Verification items for the finished model (mm, model axes). Face numbers are marked on the shaded views. Round coordinates to 2 decimals unless told otherwise and drop trailing zeros. Write each loop counter-clockwise with the first axis right and the second up, starting at its lowest first coordinate (ties: lowest second). Pieces come first, ordered by that corner, then holes.
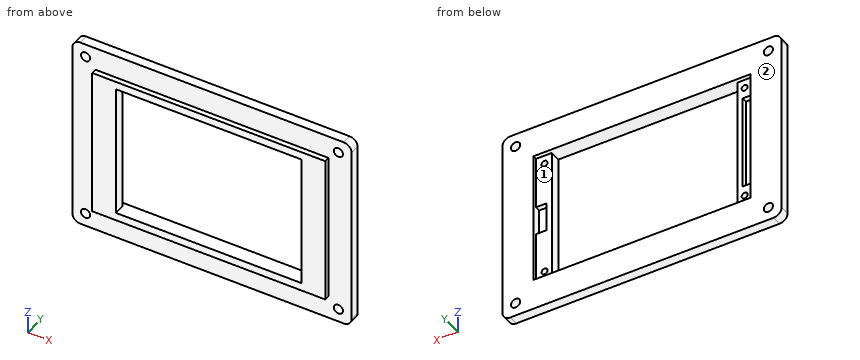
from build123d import *

# Parameters (mm, degrees)
SKETCH_1_W          = 106
SKETCH_1_H          = 74
EXTRUDE_1_DEPTH     = 5.7
SKETCH_2_W          = 70.5
SKETCH_2_H          = 50.5
CUT_EXTRUDE_1_DEPTH = 130.400502317
SKETCH_3_W          = 82.5
SKETCH_3_H          = 50.5
CUT_EXTRUDE_2_DEPTH = 1.6
SKETCH_4_W          = 4
SKETCH_4_H          = 11
SKETCH_4_H_2        = 36
CUT_EXTRUDE_3_DEPTH = 2
SKETCH_5_R          = 1.15
CUT_EXTRUDE_4_DEPTH = 3.9
CUT_EXTRUDE_START   = -5.7
SKETCH_6_W          = 131.135040239
SKETCH_6_H          = 88.560038322
SKETCH_6_W_2        = 88.5
SKETCH_6_H_2        = 56.5
CUT_EXTRUDE_5_DEPTH = 2
SKETCH_7_R          = 1.75
CUT_EXTRUDE_6_DEPTH = 130.32783923
FILLET_1_R          = 3


with BuildPart() as part:
    # Эскиз1 → Бобышка-Вытянуть1 (new body)
    with BuildSketch(Plane(origin=(0, 0, 0), x_dir=(1, 0, 0), z_dir=(0, 1, 0))):
        with Locations((53, 37)):
            Rectangle(SKETCH_1_W, SKETCH_1_H)
    extrude(amount=EXTRUDE_1_DEPTH)

    # Эскиз2 → Вырез-Вытянуть1 (cut, through all)
    with BuildSketch(Plane(origin=(0, 5.7, 0), x_dir=(1, 0, 0), z_dir=(0, 1, 0))):
        with Locations((53, 37)):
            Rectangle(SKETCH_2_W, SKETCH_2_H)
    extrude(amount=-CUT_EXTRUDE_1_DEPTH, mode=Mode.SUBTRACT)

    # Эскиз3 → Вырез-Вытянуть2 (cut)
    with BuildSketch(Plane(origin=(0, 5.7, 0), x_dir=(1, 0, 0), z_dir=(0, 1, 0))):
        with Locations((53, 37)):
            Rectangle(SKETCH_3_W, SKETCH_3_H)
    extrude(amount=-CUT_EXTRUDE_2_DEPTH, mode=Mode.SUBTRACT)

    # Эскиз4 → Вырез-Вытянуть3 (cut)
    with BuildSketch(Plane(origin=(0, 4.1, 0), x_dir=(1, 0, 0), z_dir=(0, 1, 0))):
        with Locations((92.25, 37)):
            Rectangle(SKETCH_4_W, SKETCH_4_H)
        with Locations((13.75, 37)):
            Rectangle(SKETCH_4_W, SKETCH_4_H_2)
    extrude(amount=-CUT_EXTRUDE_3_DEPTH, mode=Mode.SUBTRACT)

    # Эскиз5 → Вырез-Вытянуть4 (cut)
    with BuildSketch(Plane(origin=(0, 4.1, 0), x_dir=(1, 0, 0), z_dir=(0, 1, 0))):
        with Locations(Location((15, 59, 0), (0, 0, 270))):
            Circle(SKETCH_5_R)
        with Locations(Location((91, 59, 0), (0, 0, 270))):
            Circle(SKETCH_5_R)
        with Locations(Location((91, 15, 0), (0, 0, 270))):
            Circle(SKETCH_5_R)
        with Locations(Location((15, 15, 0), (0, 0, 270))):
            Circle(SKETCH_5_R)
    extrude(amount=-CUT_EXTRUDE_4_DEPTH, mode=Mode.SUBTRACT)

    # Эскиз6 → Вырез-Вытянуть5 (cut)
    with BuildSketch(Plane(origin=(0, 5.7, 0), x_dir=(1, 0, 0), z_dir=(0, 1, 0)).offset(CUT_EXTRUDE_START)):
        with Locations((54.065232984, 39.640866481)):
            Rectangle(SKETCH_6_W, SKETCH_6_H)
        with Locations((53, 37)):
            Rectangle(SKETCH_6_W_2, SKETCH_6_H_2, mode=Mode.SUBTRACT)
    extrude(amount=CUT_EXTRUDE_5_DEPTH, mode=Mode.SUBTRACT)

    # Эскиз7 → Вырез-Вытянуть6 (cut, through all)
    with BuildSketch(Plane.XZ.offset(-2)):
        with Locations(Location((5, -5, 0), (0, 0, 270))):
            Circle(SKETCH_7_R)
        with Locations(Location((101, -5, 0), (0, 0, 270))):
            Circle(SKETCH_7_R)
        with Locations(Location((101, -69, 0), (0, 0, 270))):
            Circle(SKETCH_7_R)
        with Locations(Location((5, -69, 0), (0, 0, 270))):
            Circle(SKETCH_7_R)
    extrude(amount=-CUT_EXTRUDE_6_DEPTH, mode=Mode.SUBTRACT)

    # Скругление1
    fillet_1_edges = [part.edges().sort_by_distance(p)[0] for p in [
        (0, 3.85, -74),
        (106, 3.85, -74),
        (106, 3.85, 0),
        (0, 3.85, 0),
    ]]
    fillet(fillet_1_edges, radius=FILLET_1_R)


solid = part.part
Q1. Sectioned sample at A-A (z = -50.5). Enter the section's corners in (x, y), plus the area to 3 significant figures.
Recorded:
outline: (0, 2) - (8.75, 2) - (8.75, 0) - (17.75, 0) - (17.75, 4.1) - (15.75, 4.1) - (15.75, 2.1) - (11.75, 2.1) - (11.75, 5.7) - (0, 5.7) - close; (88.25, 0) - (97.25, 0) - (97.25, 2) - (106, 2) - (106, 5.7) - (94.25, 5.7) - (94.25, 4.1) - (88.25, 4.1) - close
area: 140 mm2
Q2. Sectioned sample at C-C (y = 3.1). Give the number of separate pieces and of enclosed holes in the cut face, plus the area to 3 significant figures.
Recorded:
separate pieces: 1
enclosed holes: 11
area: 4,030 mm2
Q3. Release check for a two-part mould opening along X. For the marked faces 1 and 2 record: released by +X, released by -X, zero draft, split by the parting line, or undercut.
Recorded:
face 1: undercut
face 2: zero draft
Q4. Sectioned sample at D-D (z = -5). Enter the section's corners in (x, y), plus the area to 3 significant figures.
Recorded:
outline: (0, 2) - (3.25, 2) - (3.25, 5.7) - (0, 5.7) - close; (6.75, 2) - (99.25, 2) - (99.25, 5.7) - (6.75, 5.7) - close; (102.75, 2) - (106, 2) - (106, 5.7) - (102.75, 5.7) - close
area: 366 mm2
Q5. Sectioned sample at B-B (x = 79). Enter the section's corners in (y, z).
Recorded:
outline: (0, -65.25) - (2, -65.25) - (2, -74) - (5.7, -74) - (5.7, -62.25) - (0, -62.25) - close; (0, -11.75) - (5.7, -11.75) - (5.7, 0) - (2, 0) - (2, -8.75) - (0, -8.75) - close
Q6. Depth check by flat-ended pin: P1, Ø1.6, axis at x = 49.5, y = 1, coming from the +Z side; P2, Ø0.6, axis at x = 46.5, y = 1, coming from the -Z side; P3, Ø1.8, axis at x = 90.5, z = -59.5, coming from the +Y side. Enter the tip coordinate at first touch or a pass-through.
Recorded:
P1: stops at z = -8.75
P2: stops at z = -65.25
P3: stops at y = 4.1
Q7. Material ranges on line 1 along X through (y, z) = (2.45, -41); line 2 along X through (y, z) = (4.35, -5); line 3 along Z through (x, y) = (91, 1.45), recorded low to high.
Recorded:
line 1: x = 0 to 11.75, 15.75 to 17.75, 88.25 to 90.25, 94.25 to 106
line 2: x = 0 to 3.25, 6.75 to 99.25, 102.75 to 106
line 3: z = -65.25 to -60.15, -57.85 to -16.15, -13.85 to -8.75
